from build123d import *

# Parameters (mm, degrees)
SKETCH9_W           = 150
SKETCH9_H           = 40
BOSS_EXTRUDE5_DEPTH = 5
SKETCH10_R          = 10
SKETCH10_R_2        = 8
SKETCH10_R_3        = 2
CUT_EXTRUDE5_DEPTH  = 103.952823134
SKETCH11_R          = 1.7
CUT_EXTRUDE6_DEPTH  = 103.952823134
FILLET1_R           = 10


with BuildPart() as part:
    # Sketch9 → Boss-Extrude5 (new body)
    with BuildSketch(Plane(origin=(0, 0, 0), x_dir=(1, 0, 0), z_dir=(0, 1, 0))):
        with Locations((25.867654831, 0)):
            Rectangle(SKETCH9_W, SKETCH9_H)
    extrude(amount=BOSS_EXTRUDE5_DEPTH)

    # Sketch10 → Cut-Extrude5 (cut, through all)
    # profile 1 of 12: a face of its own
    with BuildSketch(Plane(origin=(0, 5, 0), x_dir=(1, 0, 0), z_dir=(0, 1, 0))):
        Circle(SKETCH10_R)
    # profile 2 of 12: a face of its own
    with BuildSketch(Plane(origin=(0, 5, 0), x_dir=(1, 0, 0), z_dir=(0, 1, 0))):
        Polygon((0.292318991, -10.661038996), (0.292318991, 11.338961004), (-30.707681009, 11.345685511), (-30.711010445, -10.656347446), align=None)
        with Locations((-13, 0)):
            Circle(SKETCH10_R_2, mode=Mode.SUBTRACT)
    # profile 3 of 12: a face of its own
    with BuildSketch(Plane(origin=(0, 5, 0), x_dir=(1, 0, 0), z_dir=(0, 1, 0))):
        with BuildLine():
            ThreePointArc((10, 0), (7.173673742, 6.966950914), (0.292318991, 9.995726567))
            Line((0.292318991, 9.995726567), (0.292318991, -9.995726567))
            ThreePointArc((0.292318991, -9.995726567), (7.173673742, -6.966950914), (10, 0))
        make_face()
    # profile 4 of 12: a face of its own
    with BuildSketch(Plane(origin=(0, 5, 0), x_dir=(1, 0, 0), z_dir=(0, 1, 0))):
        with BuildLine():
            Line((0.292318991, -9.995726567), (0.292318991, 9.995726567))
            ThreePointArc((0.292318991, 9.995726567), (-4.255176628, 9.049501194), (-7.884615385, 6.150840612))
            ThreePointArc((-7.884615385, 6.150840612), (-5.756966211, 3.396831102), (-5, 0))
            ThreePointArc((-5, 0), (-5.756966211, -3.396831102), (-7.884615385, -6.150840612))
            ThreePointArc((-7.884615385, -6.150840612), (-4.255176628, -9.049501194), (0.292318991, -9.995726567))
        make_face()
    # profile 5 of 12: a face of its own
    with BuildSketch(Plane(origin=(0, 5, 0), x_dir=(1, 0, 0), z_dir=(0, 1, 0))):
        Circle(SKETCH10_R)
    # profile 6 of 12: a face of its own
    with BuildSketch(Plane(origin=(0, 5, 0), x_dir=(1, 0, 0), z_dir=(0, 1, 0))):
        with Locations((-13, 0)):
            Circle(SKETCH10_R_2)
    # profile 7 of 12: a face of its own
    with BuildSketch(Plane(origin=(0, 5, 0), x_dir=(1, 0, 0), z_dir=(0, 1, 0))):
        Circle(SKETCH10_R)
    # profile 8 of 12: a face of its own
    with BuildSketch(Plane(origin=(0, 5, 0), x_dir=(1, 0, 0), z_dir=(0, 1, 0))):
        with Locations((-13, 0)):
            Circle(SKETCH10_R_2)
    # profile 9 of 12: a face of its own
    with BuildSketch(Plane(origin=(0, 5, 0), x_dir=(1, 0, 0), z_dir=(0, 1, 0))):
        with Locations(Location((14.5, 5, 0), (0, 0, 270))):
            Circle(SKETCH10_R_3)
    # profile 10 of 12: a face of its own
    with BuildSketch(Plane(origin=(0, 5, 0), x_dir=(1, 0, 0), z_dir=(0, 1, 0))):
        with Locations(Location((14.5, -5, 0), (0, 0, 270))):
            Circle(SKETCH10_R_3)
    # profile 11 of 12: a face of its own
    with BuildSketch(Plane(origin=(0, 5, 0), x_dir=(1, 0, 0), z_dir=(0, 1, 0))):
        with Locations(Location((-34.5, 5, 0), (0, 0, 270))):
            Circle(SKETCH10_R_3)
    # profile 12 of 12: a face of its own
    with BuildSketch(Plane(origin=(0, 5, 0), x_dir=(1, 0, 0), z_dir=(0, 1, 0))):
        with Locations(Location((-34.5, -5, 0), (0, 0, 270))):
            Circle(SKETCH10_R_3)
    extrude(amount=-CUT_EXTRUDE5_DEPTH, mode=Mode.SUBTRACT)

    # Sketch11 → Cut-Extrude6 (cut, through all)
    with BuildSketch(Plane(origin=(0, 5, 0), x_dir=(1, 0, 0), z_dir=(0, 1, 0))):
        with Locations(Location((-40, 15, 0), (0, 0, 270))):
            Circle(SKETCH11_R)
        with Locations(Location((90, 15, 0), (0, 0, 270))):
            Circle(SKETCH11_R)
        with Locations(Location((90, -15, 0), (0, 0, 270))):
            Circle(SKETCH11_R)
        with Locations(Location((-40, -15, 0), (0, 0, 270))):
            Circle(SKETCH11_R)
    extrude(amount=-CUT_EXTRUDE6_DEPTH, mode=Mode.SUBTRACT)

    # Fillet1
    fillet1_edges = [part.edges().sort_by_distance(p)[0] for p in [
        (100.867654831, 2.5, 20),
        (-49.132345169, 2.5, 20),
        (-49.132345169, 2.5, -20),
        (100.867654831, 2.5, -20),
    ]]
    fillet(fillet1_edges, radius=FILLET1_R)


solid = part.part
Here's how the part is built. I have some questions about the finished solid (model axes, mm). A direction names the side the tool comes from. Coordinates: 2 decimals unless noted, no trailing zeros. Write each loop counter-clockwise with the first axis right and the second up, starting at its lowest first coordinate (ties: lowest second). Pieces come first, ordered by that corner, then holes.
Item 1: I want a section at C-C on y = 1.65. Count the separate pieces of the cut face and the enclosed holes in it, and give its area (3 significant figures).
Item 2: If I drill on line 1 (X direction, y = 1.45, z = 14); line 2 (X direction, y = 3, z = -5); line 3 (Z direction, x = -17, y = 4.2), over which ranges is the centre line in solid material (lowest first)?
Item 3: I want a section at B-B on z = 0. Write out the boundary of the cut face in (x, y).
Item 4: If we mould it in two halves opening along Z, with no side actions, what happens to faces 3 (the flat face through (25, 0, 0)), 4 (the cylindrical face through (-36.452, 2.535, 4.566)), 5 (the cylindrical face through (97.86, 2.54, -17.15))? For each: +Z half, -Z half, draft (parallel to the pull), parting line (faces both ways), or undercut.
Item 5: On a 3-axis mill with a long thin cutter (end or side, diameter ignored), from which of +Z, -Z, +X, -X, +Y, -Y can I reach the whole of each face in a straight line? I mean faces 1 (the cylindrical face through (10, 3, 0)), 2 (the cylindrical face through (97.86, 2.54, 17.15)). Say none if no direction works.
Item 6: Will this pin go through, and if not, where does the flat tip stop? pin 1 (6.5 mm diameter, centred on x = 14.5, z = 5, fed in from -Y).
Item 7: I want a section at D-D on z = 15. Write out the boundary of the cut face in (x, y).
Item 8: I want a section at A-A on x = 14.5. Write out the boundary of the cut face in (y, z).
Findings below:
1. separate pieces: 1
1. enclosed holes: 9
1. area: 4,990 mm2
2. line 1: x = -48.3 to -41.37, -38.63 to 88.63, 91.37 to 100.03
2. line 2: x = -49.13 to -36.5, -32.5 to -30.71, 8.66 to 12.5, 16.5 to 100.87
2. line 3: z = -20 to -11.34, 10.66 to 20
3. outline: (-49.13, 0) - (-30.71, 0) - (-30.71, 5) - (-49.13, 5) - close; (10, 0) - (100.87, 0) - (100.87, 5) - (10, 5) - close
4. face 3: draft
4. face 4: undercut
4. face 5: -Z half
5. face 1: +Y, -Y
5. face 2: +Z, +X, +Y, -Y
6. pin 1: stops at y = 0
7. outline: (-47.79, 0) - (-41.7, 0) - (-41.7, 5) - (-47.79, 5) - close; (-38.3, 0) - (88.3, 0) - (88.3, 5) - (-38.3, 5) - close; (91.7, 0) - (99.53, 0) - (99.53, 5) - (91.7, 5) - close
8. outline: (0, -20) - (5, -20) - (5, -7) - (0, -7) - close; (0, -3) - (5, -3) - (5, 3) - (0, 3) - close; (0, 7) - (5, 7) - (5, 20) - (0, 20) - close
